Can you work these out from the model? Positions are in its coordinate system, mm. Face numbers are marked on the shaded views. A direction names the side the tool comes from. Coordinates: 2 decimals unless noted, no trailing zeros. Order: outer loops, then holes, each group sorted by start corner. A loop starts at its lowest first (then second) coordinate and runs counter-clockwise, first axis right, second up. Notation, with made-up numbers: (-4.75, 38.5) -> (24.25, 38.5) arc R19 cw to (24.25, 53.5) -> close; hole circle Ø10 at (83.5, 71.5). An arc over 180 degrees is marked (long way). Answer as CSV lines item,"result".
from build123d import *

# Parameters (mm, degrees)
F1_DEPTH  = 1.7
F2_W      = 22.915563779
F2_H      = 18.9440016984
F3_DEPTH  = 3
F4_W      = 9
F4_H      = 5
F5_DEPTH  = 2
F6_W      = 2.8090730775
F6_H      = 6.5048590768
F6_W_2    = 0.9965691715
F6_H_2    = 2.0780880004
F6_W_3    = 2.6543419808
F6_H_3    = 1.4811633155
F6_W_4    = 1.4437921345
F6_H_4    = 2.3924442939
F6_W_5    = 0.7371641695
F6_H_5    = 1.757067279
F6_W_6    = 0.7299780846
F6_H_6    = 1.4931405894
F6_R      = 2.3137841174
F7_DEPTH  = 1.5
F8_W      = 7
F8_H      = 4
F9_DEPTH  = 3
F10_W     = 6.5
F10_H     = 2.3
F10_H_2   = 1.7
F10_H_3   = 2.5
F11_DEPTH = 1.5
F12_R     = 3.15
F13_DEPTH = 8


with BuildPart() as f1:
    # F0 (on Top) → F1 (new body)
    with BuildSketch(Plane.XY):
        Polygon((-26, 20), (-26, 0), (0, 0), (0, 10), (3, 10), (3, 20), align=None)
    extrude(amount=F1_DEPTH)

    # F2 (on face) → F3 (join)
    with BuildSketch(Plane.XY.offset(1.7)):
        with Locations((-12.8477554535, 9.9514690519)):
            Rectangle(F2_W, F2_H)
    extrude(amount=F3_DEPTH)

    # F4 (on face) → F5 (join)
    with BuildSketch(Plane(origin=(0, 0, 0), x_dir=(1, 0, 0), z_dir=(0, 0, -1))):
        with Locations((-9.5, -15.5)):
            Rectangle(F4_W, F4_H)
    extrude(amount=F5_DEPTH)

    # F6 (on face) → F7 (join)
    with BuildSketch(Plane(origin=(0, 0, 0), x_dir=(1, 0, 0), z_dir=(0, 0, -1))):
        with Locations((-3.8609959884, -5.2312271437)):
            Rectangle(F6_W, F6_H)
        with Locations((-15.6953232363, -13.6427599937)):
            Rectangle(F6_W_2, F6_H_2)
        with Locations((-18.9768830314, -12.8015675582)):
            Rectangle(F6_W_3, F6_H_3)
        with Locations((-12.4409804121, -3.1250810716)):
            Rectangle(F6_W_4, F6_H_4)
        with Locations((-24.7127972543, -2.3718061275)):
            Rectangle(F6_W_5, F6_H_5)
        with Locations((-24.7733462602, -4.7515959013)):
            Rectangle(F6_W_6, F6_H_6)
        with Locations((-19.4019284099, -2.9428394046)):
            Circle(F6_R)
    extrude(amount=F7_DEPTH)

    # F8 (on face) → F9 (join)
    with BuildSketch(Plane(origin=(0, 0, 0), x_dir=(1, 0, 0), z_dir=(0, 0, -1))):
        with Locations((-19.5, -18)):
            Rectangle(F8_W, F8_H)
    extrude(amount=F9_DEPTH)

    # F10 (on face) → F11 (join)
    with BuildSketch(Plane.YZ.offset(3)):
        with Locations((15, -1.15)):
            Rectangle(F10_W, F10_H)
        with Locations((15, 0.85)):
            Rectangle(F10_W, F10_H_2)
        with Locations((15, 2.95)):
            Rectangle(F10_W, F10_H_3)
    extrude(amount=F11_DEPTH)

    # F12 (on face) → F13 (join)
    with BuildSketch(Plane.YZ.offset(4.5)):
        with Locations((15, 0.95)):
            Circle(F12_R)
    extrude(amount=F13_DEPTH)


solid = f1.part
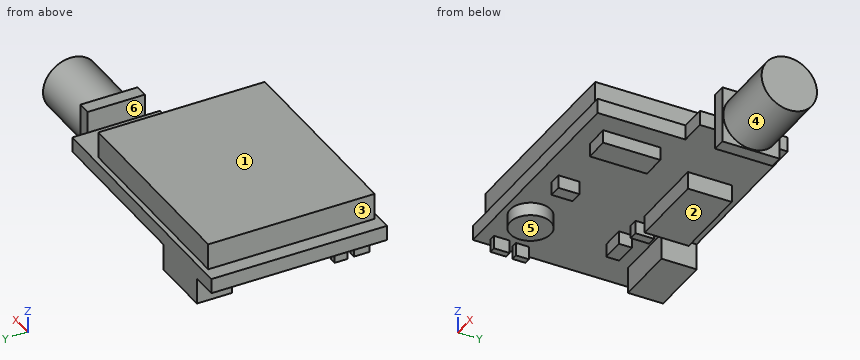
Q1. We'd pull the mould along X, two halves only. Please class the marked faces 1, 2 and 3: pulls with the +X half, pulls with the -X half, needs draft (parallel to the pull), parting line crosses it, or undercut.
Solution:
face 1,"needs draft"
face 2,"undercut"
face 3,"pulls with the -X half"
Q2. Imagine slicing it at D-D (x = 9). List the corners of the cut face in (y, z) for me, and give its area (3 significant figures).
Solution:
outline,"circle Ø6.3 at (15, 0.95)"
area,"31.2 mm2"
Q3. If I drill on line 1 (X direction, y = 16.5, z = -1.25); line 2 (X direction, y = 15.25, z = 3.75); line 3 (X direction, y = 3.75, z = -1), over which ranges is the centre line in solid material (lowest first)?
Solution:
line 1,"-23 to -16, -14 to -5, 3 to 12.5"
line 2,"-24.31 to -1.39, 3 to 12.5"
line 3,"-21.57 to -17.23, -13.16 to -11.72, -5.27 to -2.46"
Q4. Imagine slicing it at C-C (y = 7). List the corners of the cut face in (x, z) for me, and give its area (3 significant figures).
Solution:
outline,"(-26, 0) -> (-5.27, 0) -> (-5.27, -1.5) -> (-2.46, -1.5) -> (-2.46, 0) -> (0, 0) -> (0, 1.7) -> (-1.39, 1.7) -> (-1.39, 4.7) -> (-24.31, 4.7) -> (-24.31, 1.7) -> (-26, 1.7) -> close"
area,"117 mm2"
Q5. Imagine slicing it at A-A (y = 9.25). List the corners of the cut face in (x, z) for me.
Solution:
outline,"(-26, 0) -> (0, 0) -> (0, 1.7) -> (-1.39, 1.7) -> (-1.39, 4.7) -> (-24.31, 4.7) -> (-24.31, 1.7) -> (-26, 1.7) -> close"
Q6. Imagine slicing it at B-B (z = 0.95). List the corners of the cut face in (x, y) for me, and give its area (3 significant figures).
Solution:
outline,"(-26, 0) -> (0, 0) -> (0, 10) -> (3, 10) -> (3, 11.75) -> (4.5, 11.75) -> (4.5, 11.85) -> (12.5, 11.85) -> (12.5, 18.15) -> (4.5, 18.15) -> (4.5, 18.25) -> (3, 18.25) -> (3, 20) -> (-26, 20) -> close"
area,"610 mm2"
Q7. For P1, Ø1.5, axis at x = 6, y = 12, coming from the -Z side; P2, Ø0.7, axis at y = 13, z = -0.5, coming from the -X side; P3, Ø1.6, axis at x = -13, z = -1, coming from the -Y side; P4, Ø1, axis at x = -7, z = 1.5, coming from the -Y side, each with a flat end and sliding along its axis, tell me the tip position at first contact or that it passes through.
Solution:
P1,"z = -1.25"
P2,"x = -20.3"
P3,"y = 1.93"
P4,"y = 0"
Q8. Which directions (+Z, -Z, +X, -X, +Y, -Y) give clear straight access to the entire face, cutting with the end or side of a thin tool? Please do the marked faces 4, 5 and 6.
Solution:
face 4,"+X"
face 5,"-Z, +X, -X, -Y"
face 6,"+Z, +Y, -Y"
